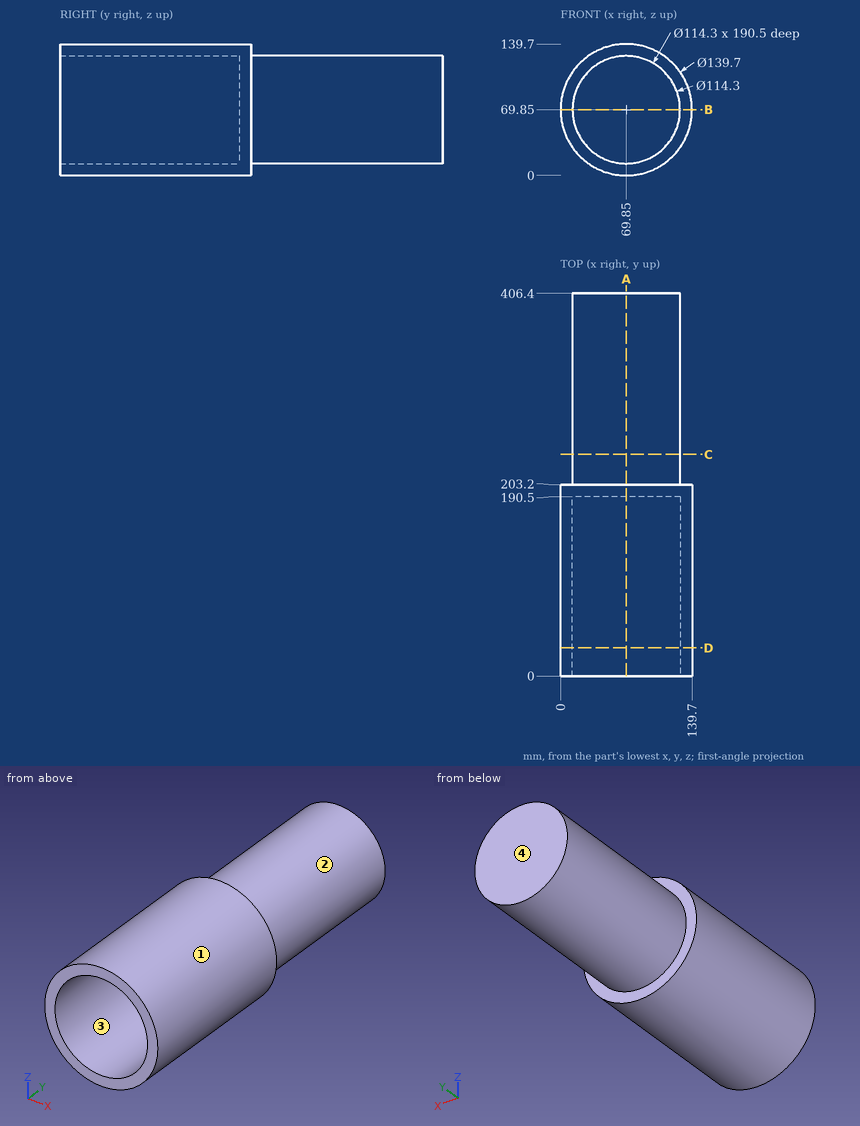
The figure shows three views and two pictorial views of one solid part (mm, origin at its lowest corner). Answer the questions. A direction names the side the tool comes from. Give positions to 0.01 mm unless a question says otherwise; leave off trailing zeros. Write each loop counter-clockwise with the first axis right and the second up, starting at its lowest first coordinate (ties: lowest second). Pieces come first, ordered by that corner, then holes. Notation, with made-up numbers: (68, 30) - (123, 30) arc R22 cw to (123, 67) - close; hole circle Ø10 at (-37.5, -10). An arc over 180 degrees is marked (long way). Use one line per item in the form item = value. Start each with the question number.
1) Find section B-B on z = 69.85. Determine the outline of the cut face in (x, y).
2) The mould has two halves that part along Y. Classify the marked faces 3 and 4: pulls with the +Y half, pulls with the -Y half, needs draft (parallel to the pull), parting line crosses it, or undercut.
3) Consider line 1 along Z through (x, y) = (69, 128); line 2 along Y through (x, z) = (81, 133). Determine where each line is inside the solid, lowest interval first. Write a range as from..to.
4) A tool of negligible diameter and unlimited length cuts with its end or side. For the marked faces 1 and 2, from which of +Z, -Z, +X, -X, +Y, -Y can it reach the whole face along a straight path? Write none if from no direction.
5) Find section A-A on x = 69.85. Determine the outline of the cut face in (y, z), plus the area to 3 significant figures.
6) Flat-ended cylindrical pins translate along their axes: pin 1 Ø3 at (x, z) = (60.5, 36.5) entering from -Y; pin 2 Ø8 at (x, z) = (32.5, 117) entering from +Y; pin 3 Ø6 at (y, z) = (105, 55.5) entering from +X; pin 4 Ø1 at (y, z) = (163.5, 124.5) entering from +X. Find the tip coordinate at first contact, or state that the pin passes through.
7) Find section D-D on y = 30. Determine the outline of the cut face in (x, z), plus the area to 3 significant figures.
8) Find section C-C on y = 235.5. Determine the outline of the cut face in (x, z).
Geometry results:
q1.outline = (0, 0) - (12.7, 0) - (12.7, 190.5) - (127, 190.5) - (127, 0) - (139.7, 0) - (139.7, 203.2) - (127, 203.2) - (127, 406.4) - (12.7, 406.4) - (12.7, 203.2) - (0, 203.2) - close
q2.face_3 = needs draft
q2.face_4 = pulls with the +Y half
q3.line_1 = 0.01..12.71, 126.99..139.69
q3.line_2 = 0..203.2
q4.face_1 = +Y, -Y
q4.face_2 = +Y
q5.outline = (0, 0) - (203.2, 0) - (203.2, 12.7) - (406.4, 12.7) - (406.4, 127) - (203.2, 127) - (203.2, 139.7) - (0, 139.7) - (0, 127) - (190.5, 127) - (190.5, 12.7) - (0, 12.7) - close
q5.area = 29,800 mm2
q6.pin_1 = 190.5
q6.pin_2 = 406.4
q6.pin_3 = 138.77
q6.pin_4 = 113.97
q7.outline = circle Ø139.7 at (69.85, 69.85); hole circle Ø114.3 at (69.85, 69.85)
q7.area = 5,070 mm2
q8.outline = circle Ø114.3 at (69.85, 69.85)
